Verification items for the finished model (mm, model axes). Face numbers are marked on the shaded views. A direction names the side the tool comes from. Coordinates: 2 decimals unless noted, no trailing zeros. Order: outer loops, then holes, each group sorted by start corner. A loop starts at its lowest first (then second) coordinate and runs counter-clockwise, first axis right, second up. Notation, with made-up numbers: M 76.5,53 L 109.5,53 A30 cw 109.5,80 Z; hole C 87,24 d4. An arc over 180 degrees is marked long. Return JSON: item names as keys, results as strings. Group by question number.
1. Gauge pin test, flat ends, axial feed: pin 1 (2 mm diameter, centred on x = 1.86, y = 3.96, fed in from +Z); pin 2 (0.9 mm diameter, centred on y = 0, z = 2, fed in from +X); pin 3 (1.5 mm diameter, centred on x = -3.5, z = 2.5, fed in from -Y); pin 4 (1.5 mm diameter, centred on x = 11, z = 3, fed in from -Y). Record the tip position at first contact, or that the pin passes through.
2. Set-up check for the marked faces 1 and 2: record each of +Z, -Z, +X, -X, +Y, -Y from which the full face is reachable in a straight line by a thin tool's end or side.
3. Section check C-C, the plane y = -5.5. Record the cut outline in (x, z), plus the area to 3 significant figures.
4. Section check A-A, the plane z = 2.5. Give the number of separate pieces and of enclosed holes in the cut face, plus the area to 3 significant figures.
5. Section check D-D, the plane x = -1.5. Record the cut outline in (y, z), plus the area to 3 significant figures.
6. Section check B-B, the plane x = -13.25. Record the cut outline in (y, z), plus the area to 3 significant figures.
7. Material ranges on line 1 along X through (y, z) = (0.5, 2.3); line 2 along X through (y, z) = (-3.5, 2.45); line 3 along Y through (x, z) = (-7.75, 2.1), recorded low to high.
```python
from build123d import *

# Parameters (mm, degrees)
SKETCH1_W           = 28
SKETCH1_H           = 18
BOSS_EXTRUDE1_DEPTH = 1
SKETCH2_W           = 1.4
SKETCH2_H           = 1.4
BOSS_EXTRUDE3_DEPTH = 3
SKETCH3_R           = 1.25
CUT_EXTRUDE1_DEPTH  = 10


with BuildPart() as part:
    # Sketch1 → Boss-Extrude1 (new body)
    with BuildSketch(Plane.XY):
        with Locations((-1.236641221, -1.241221374)):
            Rectangle(SKETCH1_W, SKETCH1_H)
    extrude(amount=BOSS_EXTRUDE1_DEPTH)

    # Sketch2 → Boss-Extrude3 (add)
    with BuildSketch(Plane.XY.offset(1)):
        with Locations((10.763358779, -2.241221374)):
            Rectangle(SKETCH2_W, SKETCH2_H)
        with Locations((-13.236641221, -2.241221374)):
            Rectangle(SKETCH2_W, SKETCH2_H)
        Polygon((-8.112377153, 6.458778626), (5.63909471, 6.458778626), (7.463358779, 4.634514557), (7.463358779, -8.941221374), (-9.936641221, -8.941221374), (-9.936641221, 4.634514557), align=None)
    extrude(amount=BOSS_EXTRUDE3_DEPTH)

    # Sketch3 → Cut-Extrude1 (cut)
    with BuildSketch(Plane.XY.offset(4)):
        with Locations((-7.436641221, 3.958778626)):
            Circle(SKETCH3_R)
        with Locations((-4.336641221, 3.958778626)):
            Circle(SKETCH3_R)
        with Locations((-1.236641221, 3.958778626)):
            Circle(SKETCH3_R)
        with Locations((1.863358779, 3.958778626)):
            Circle(SKETCH3_R)
        with Locations((4.963358779, 3.958778626)):
            Circle(SKETCH3_R)
        with Locations((-4.336641221, 0.492111959)):
            Circle(SKETCH3_R)
        with Locations((-1.236641221, 0.492111959)):
            Circle(SKETCH3_R)
        with Locations((1.863358779, 0.492111959)):
            Circle(SKETCH3_R)
        with Locations((4.963358779, 0.492111959)):
            Circle(SKETCH3_R)
        with Locations((-4.336641221, -2.974554707)):
            Circle(SKETCH3_R)
        with Locations((-1.236641221, -2.974554707)):
            Circle(SKETCH3_R)
        with Locations((1.863358779, -2.974554707)):
            Circle(SKETCH3_R)
        with Locations((4.963358779, -2.974554707)):
            Circle(SKETCH3_R)
        with Locations((-4.336641221, -6.441221374)):
            Circle(SKETCH3_R)
        with Locations((-1.236641221, -6.441221374)):
            Circle(SKETCH3_R)
        with Locations((1.863358779, -6.441221374)):
            Circle(SKETCH3_R)
        with Locations((4.963358779, -6.441221374)):
            Circle(SKETCH3_R)
        with Locations((-7.436641221, 0.492111959)):
            Circle(SKETCH3_R)
        with Locations((-7.436641221, -2.974554707)):
            Circle(SKETCH3_R)
        with Locations((-7.436641221, -6.441221374)):
            Circle(SKETCH3_R)
    extrude(amount=-CUT_EXTRUDE1_DEPTH, mode=Mode.SUBTRACT)


solid = part.part
```
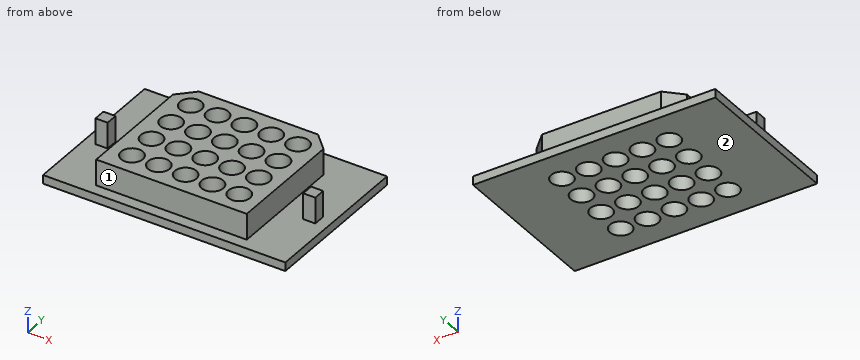
Answers follow:
{
 "1": {"pin 1": "through", "pin 2": "x = 7.46", "pin 3": "y = -8.94", "pin 4": "y = -2.94"},
 "2": {"face 1": "+Z, +X, -X, -Y", "face 2": "-Z, +X, -X, +Y, -Y"},
 "3": {"outline": "M -15.24,0 L -8.26,0 L -8.26,4 L -9.94,4 L -9.94,1 L -15.24,1 Z; M -6.61,0 L -5.16,0 L -5.16,4 L -6.61,4 Z; M -3.51,0 L -2.06,0 L -2.06,4 L -3.51,4 Z; M -0.41,0 L 1.04,0 L 1.04,4 L -0.41,4 Z; M 2.69,0 L 4.14,0 L 4.14,4 L 2.69,4 Z; M 5.79,0 L 12.76,0 L 12.76,1 L 7.46,1 L 7.46,4 L 5.79,4 Z", "area": "47.3 mm^2"},
 "4": {"separate pieces": "3", "enclosed holes": "20", "area": "170 mm^2"},
 "5": {"outline": "M -10.24,0 L -7.66,0 L -7.66,4 L -8.94,4 L -8.94,1 L -10.24,1 Z; M -5.22,0 L -4.2,0 L -4.2,4 L -5.22,4 Z; M -1.75,0 L -0.73,0 L -0.73,4 L -1.75,4 Z; M 1.71,0 L 2.74,0 L 2.74,4 L 1.71,4 Z; M 5.18,0 L 7.76,0 L 7.76,1 L 6.46,1 L 6.46,4 L 5.18,4 Z", "area": "25.1 mm^2"},
 "6": {"outline": "M -10.24,0 L 7.76,0 L 7.76,1 L -1.54,1 L -1.54,4 L -2.94,4 L -2.94,1 L -10.24,1 Z", "area": "22.2 mm^2"},
 "7": {"line 1": "-9.94 to -8.69, -6.19 to -5.59, -3.09 to -2.49, 0.01 to 0.61, 3.11 to 3.71, 6.21 to 7.46", "line 2": "-9.94 to -8.57, -6.3 to -5.47, -3.2 to -2.37, -0.1 to 0.73, 3 to 3.83, 6.1 to 7.46", "line 3": "-8.94 to -7.65, -5.23 to -4.18, -1.76 to -0.72, 1.7 to 2.75, 5.17 to 6.46"}
}
